```python
from build123d import *

# Parameters (mm, degrees)
SKETCH2_R           = 5
BOSS_EXTRUDE3_DEPTH = 4
FILLET3_R           = 10
SKETCH5_R           = 5
CUT_EXTRUDE3_DEPTH  = 4


with BuildPart() as part:
    # Sketch2 → Boss-Extrude3 (new body)
    # profile 1 of 2: a face of its own
    with BuildSketch(Plane.XY):
        with BuildLine():
            ThreePointArc((14.959120664, 109.549078448), (26.821882285, 103.16737517), (20.440179007, 91.304613549))
            Line((20.440179007, 91.304613549), (-115.084548239, 50.589857539))
            Line((-115.084548239, 50.589857539), (-77.965074882, 13.470384182))
            ThreePointArc((-77.965074882, 13.470384182), (-77.965074882, 0), (-91.435459064, 0))
            Line((-91.435459064, 0), (-151.097343154, 59.661884091))
            Line((-151.097343154, 59.661884091), (14.959120664, 109.549078448))
        make_face()
        with Locations((17.699649835, 100.426845999)):
            Circle(SKETCH2_R, mode=Mode.SUBTRACT)
        with Locations((-84.700266973, 6.735192091)):
            Circle(SKETCH2_R, mode=Mode.SUBTRACT)
    # profile 2 of 2: a face of its own
    with BuildSketch(Plane.XY):
        Polygon((-94.417910685, 29.923219984), (-87.300193609, 22.805502909), (-15.947819408, 80.372818981), (-41.344385101, 72.743104488), align=None)
    extrude(amount=BOSS_EXTRUDE3_DEPTH)

    # Fillet3
    fillet3_edges = [part.edges().sort_by_distance(p)[0] for p in [
        (-151.097343154, 59.661884091, 2),
    ]]
    fillet(fillet3_edges, radius=FILLET3_R)

    # Sketch5 → Cut-Extrude3 (cut)
    with BuildSketch(Plane.XY.offset(4)):
        with Locations((-116.663330616, 60.061105539)):
            Circle(SKETCH5_R)
        with Locations((-67.81988128, 74.734805039)):
            Circle(SKETCH5_R)
    extrude(amount=-CUT_EXTRUDE3_DEPTH, mode=Mode.SUBTRACT)


solid = part.part
```
Model file for the job. Use its own axes, mm. A direction names the side the tool comes from. Coordinates: 2 decimals unless noted, no trailing zeros. Order: outer loops, then holes, each group sorted by start corner. A loop starts at its lowest first (then second) coordinate and runs counter-clockwise, first axis right, second up. Notation, with made-up numbers: (-23.75, 77) - (29.25, 77) arc R10 cw to (29.25, 92) - close; hole circle Ø11 at (4, -38). An arc over 180 degrees is marked (long way). Return JSON: item names as keys, results as strings. Group by question number.
1) Saw through at D-D, the plane y = 88. Write the cut outline in (x, z), plus the area to 3 significant figures.
2) Tool access for faces 1 (the flat face through (-61.1, 86.7, 2)), 2 (the flat face through (-52.12, 51.19, 1.97)), 3 (the flat face through (-77.7, 61.82, 1.97)): list every direction of +Z, -Z, +X, -X, +Y, -Y with a clear straight run to the whole face (end or side of a thin tool).
3) Mould opens along X. For faces 4 (the flat face through (-104.896, 40.401, 1.972)), 5 (the flat face through (-63.4, 66.4, 0)), 6 (the flat face through (2.501, 85.915, 1.972)) say: released by +X, released by -X, zero draft, split by the parting line, or undercut.
4) Saw through at A-A, the plane y = 57.5. Write the cut outline in (x, z), plus the area to 3 significant figures.
5) Probe line 1 (Y direction, x = 13.5, z = 2.7); line 2 (Y direction, x = -114.5, z = 0.95); line 3 (Y direction, x = -45, z = 3.1). List the from-to ranges inside material, lowest first. Write a range as from..to.
6) Saw through at B-B, the plane x = -82.5. Write the cut outline in (y, z), plus the area to 3 significant figures.
7) Flat gauge pins, fed straight in: P1, Ø8, axis at x = -116.66, y = 60.06, coming from the +Z side; P2, Ø11.5, axis at x = -84.7, y = 6.74, coming from the +Z side; P3, Ø2, axis at y = 20, z = 1, coming from the +X side. Where does each tip first touch, or does it go through?
8) Saw through at C-C, the plane z = 1.7. Count the separate pieces of the cut face and the enclosed holes in it, plus the area to 3 significant figures.
Values found:
{
 "1": {"outline": "(-56.77, 0) - (9.44, 0) - (9.44, 4) - (-56.77, 4) - close", "area": "265 mm²"},
 "2": {"face 1": "+Z, -Z, -X, +Y", "face 2": "+Z, -Z, +X", "face 3": "+Z, -Z"},
 "3": {"face 4": "undercut", "face 5": "zero draft", "face 6": "released by +X"},
 "4": {"outline": "(-141.85, 0) - (-120.96, 0) - (-120.96, 4) - (-141.85, 4) - close; (-112.37, 0) - (-92.08, 0) - (-92.08, 4) - (-112.37, 4) - close; (-60.24, 0) - (-44.3, 0) - (-44.3, 4) - (-60.24, 4) - close", "area": "228 mm²"},
 "5": {"line 1": "y = 89.22..97.71, 103.14..109.11", "line 2": "y = 23.06..50.01, 50.77..55.55, 64.57..70.66", "line 3": "y = 56.93..69.79, 71.64..91.54"},
 "6": {"outline": "(-2.53, 0) - (2.25, 0) - (2.25, 4) - (-2.53, 4) - close; (11.23, 0) - (18.01, 0) - (18.01, 4) - (11.23, 4) - close; (26.68, 0) - (39.54, 0) - (39.54, 4) - (26.68, 4) - close; (60.38, 0) - (80.27, 0) - (80.27, 4) - (60.38, 4) - close", "area": "177 mm²"},
 "7": {"P1": "passes through", "P2": "stops at z = 4", "P3": "stops at x = -83.49"},
 "8": {"separate pieces": "1", "enclosed holes": "5", "area": "5,010 mm²"}
}
